Autodesk Inventor part; units mm, degrees
ref_plane "YZ Plane" through (0, 0, 0) normal (1, 0, 0) x (0, 1, 0)
ref_plane "XZ Plane" through (0, 0, 0) normal (0, 1, 0) x (-1, 0, 0)
ref_plane "XY Plane" through (0, 0, 0) normal (0, 0, 1) x (1, 0, 0)
sketch "Sketch1" plane through (0, 0, 0) normal (0, 1, 0) x (-1, 0, 0)
  line L0 (-10, 25) -> (10, 25)
  line L1 (10, 25) -> (10, -25)
  line L2 (10, -25) -> (-10, -25)
  line L3 (-10, -25) -> (-10, 25)
  line L4 (-10, 25) -> (10, -25) construction
  line L5 (10, 25) -> (-10, -25) construction
  point P0 (0, 0)
  dimension "d2" = 50
  dimension "d3" = 20
extrude "Extrusion1" add sketch "Sketch1" along normal blind 9
sketch "Sketch2" plane through (0, 0, 0) normal (0, -1, 0) x (1, 0, 0)
  point P0 (0, 0)
hole "Hole1" at (0, 0, 0) direction (0, 1, 0) diameter 5.5 depth 5 tip angle 118
properties part number "SP44V1 Tope Hierro"
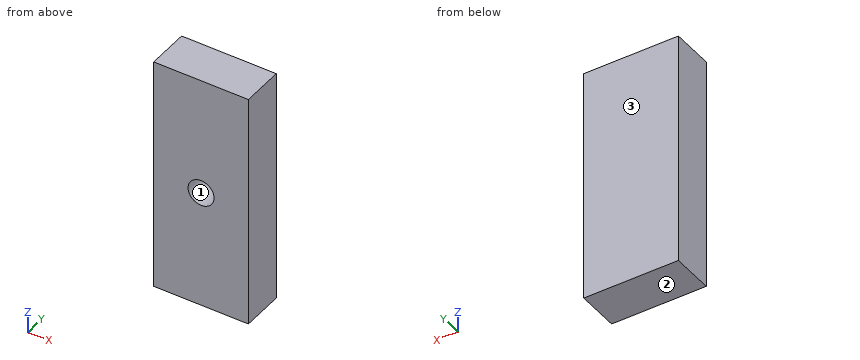
Here's how the part is built. I have some questions about the finished solid (model axes, mm). Face numbers are marked on the shaded views. Coordinates: 2 decimals unless noted, no trailing zeros. Loops run counter-clockwise (first coordinate to the right, second up) from the corner with the lowest first, then second, coordinate; pieces in that order, holes last.
1. If we mould it in two halves opening along Z, with no side actions, what happens to the marked faces 1, 2 and 3? For each: pulls with the +Z half, pulls with the -Z half, needs draft (parallel to the pull), parting line crosses it, or undercut.
2. Imagine slicing it at A-A, the plane y = 3.5. Please give me the cut outline in (x, z), and give its area (3 significant figures).
3. I need wall thicknesses on L1, parallel to X at y = 2.45, z = 0; L2, parallel to Z at x = -0.25, y = 1.5; L3, parallel to X at y = 1, z = -2.5. Which ranges of each line are inside material? Lowest first, please.
Taken from the geometry:
1. face 1: undercut
1. face 2: pulls with the -Z half
1. face 3: needs draft
2. outline: (-10, -25) - (10, -25) - (10, 25) - (-10, 25) - close; hole circle Ø5.5 at (0, 0)
2. area: 976 mm2
3. L1: x = -10 to -2.75, 2.75 to 10
3. L2: z = -25 to -2.74, 2.74 to 25
3. L3: x = -10 to -1.15, 1.15 to 10
